Part print with two shaded views. Sizes in mm from the minimum x, y, z corner. A direction names the side the tool comes from. Round coordinates to 2 decimals unless told otherwise and drop trailing zeros. Loops run counter-clockwise (first coordinate to the right, second up) from the corner with the lowest first, then second, coordinate; pieces in that order, holes last. Notation, with made-up numbers: M 3,53 L 31,53 A26 cw 31,84 Z; hole C -20,46 d3. An arc over 180 degrees is marked long. Answer as CSV lines item,"result". Start each with the question number.
Item 1: Band-saw the part on D-D (x = 24.5). Give the cut face in (y, z), and give its area (3 significant figures).
Item 2: Band-saw the part on A-A (x = 2.5). Give the cut face in (y, z), and give its area (3 significant figures).
Item 3: Which spindle directions (+Z, -Z, +X, -X, +Y, -Y) get a long thin tool onto all of the face, cutting with end or side? Do the marked faces 1, 2 and 3. Say none if no direction does.
Item 4: Band-saw the part on C-C (y = 19). Give the cut face in (x, z), and give its area (3 significant figures).
Item 5: Wall check: line 1 (X direction, y = 33.5, z = 0.65); line 2 (Y direction, x = 77.5, z = 0.5); line 3 (Z direction, x = 38, y = 34). Give the ranges that are in metal, low to high.
Item 6: Band-saw the part on B-B (y = 33.5). Give the cut face in (x, z), and give its area (3 significant figures).
Item 7: Drop flat-ended pins along their axis: pin 1 Ø5 at (x, z) = (48, 6.5) entering from -Y; pin 2 Ø5 at (y, z) = (31, 7) entering from -X; pin 3 Ø1.5 at (y, z) = (28, 3) entering from +X. Give the stop position or say it passes through.
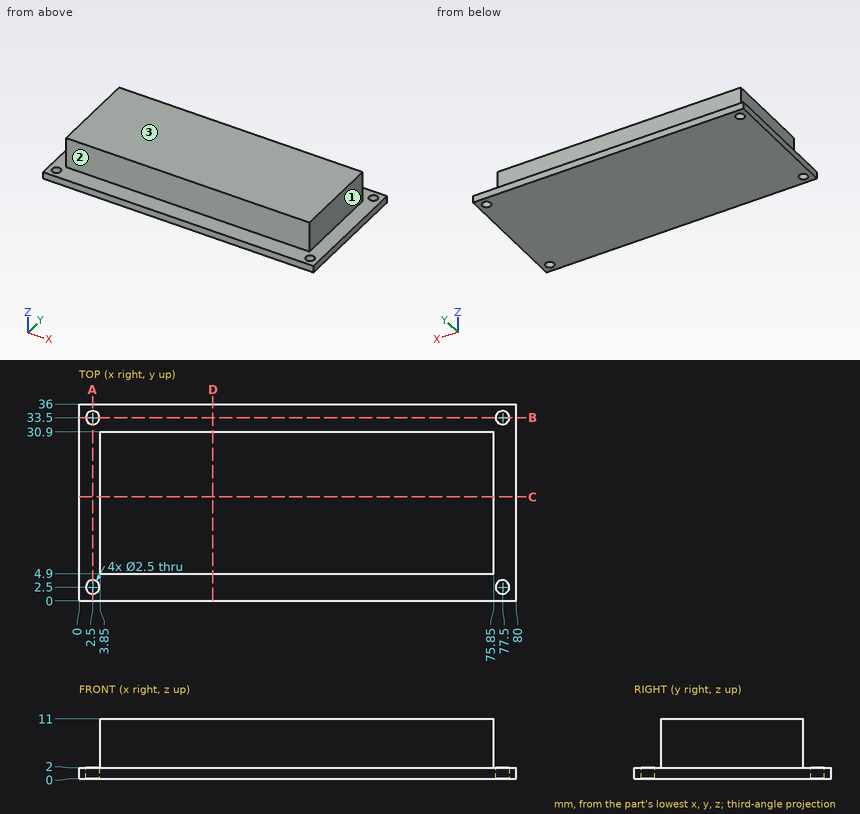
Answer block:
1,outline,"M 0,0 L 36,0 L 36,2 L 30.9,2 L 30.9,11 L 4.9,11 L 4.9,2 L 0,2 Z"
1,area,"306 mm^2"
2,outline,"M 0,0 L 1.25,0 L 1.25,2 L 0,2 Z; M 3.75,0 L 32.25,0 L 32.25,2 L 3.75,2 Z; M 34.75,0 L 36,0 L 36,2 L 34.75,2 Z"
2,area,"62.0 mm^2"
3,face 1,"+Z, +X, +Y, -Y"
3,face 2,"+Z, +X, -X, -Y"
3,face 3,"+Z, +X, -X, +Y, -Y"
4,outline,"M 0,0 L 80,0 L 80,2 L 75.85,2 L 75.85,11 L 3.85,11 L 3.85,2 L 0,2 Z"
4,area,"808 mm^2"
5,line 1,"x = 0 to 1.25, 3.75 to 76.25, 78.75 to 80"
5,line 2,"y = 0 to 1.25, 3.75 to 32.25, 34.75 to 36"
5,line 3,"z = 0 to 2"
6,outline,"M 0,0 L 1.25,0 L 1.25,2 L 0,2 Z; M 3.75,0 L 76.25,0 L 76.25,2 L 3.75,2 Z; M 78.75,0 L 80,0 L 80,2 L 78.75,2 Z"
6,area,"150 mm^2"
7,pin 1,"stops at y = 4.9"
7,pin 2,"stops at x = 3.85"
7,pin 3,"stops at x = 75.85"
